Could you check a few things on this drawing? It's one solid part, dimensions in mm from its lowest x, y, z. Give positions to 0.01 mm unless a question says otherwise; leave off trailing zeros. Write each loop counter-clockwise with the first axis right and the second up, starting at its lowest first coordinate (ties: lowest second). Pieces come first, ordered by that corner, then holes. Notation, with made-up numbers: M -26,9.25 L 23,9.25 A18 cw 23,27.25 Z; hole C 42.5,88 d8. An arc over 180 degrees is marked long. Write each question's results on one line, items separated by ' | '.
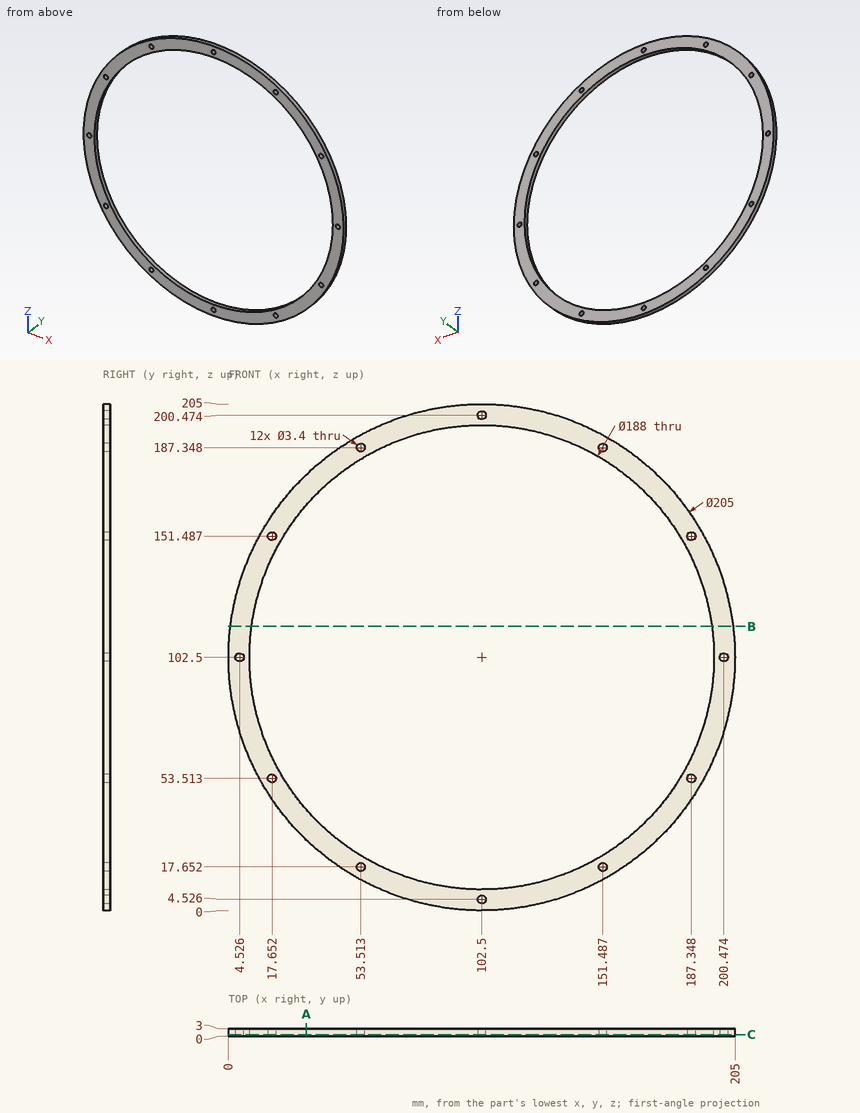
Item 1: I want a section at C-C, the plane y = 0.55. Give the number of separate pieces and of enclosed holes in the cut face, and give its area (3 significant figures).
Geometry says:
separate pieces: 1 | enclosed holes: 13 | area: 5,140 mm2
Item 2: If I drill on line 1 (X direction, y = 2.65, z = 102); line 2 (Z direction, x = 101.5, y = 1.8) (3 decimals); line 3 (X direction, y = 1.35, z = 16.5), over which ranges is the centre line in solid material (lowest first)? Write a range as from..to.
Geometry says:
line 1: x = 0..2.9, 6.15..8.5, 196.5..198.85, 202.1..205 | line 2: z = 0.005..3.151, 5.901..8.505, 196.495..199.099, 201.849..204.995 | line 3: x = 46.73..52.26, 54.76..64.55, 140.45..150.24, 152.74..158.27
Item 3: I want a section at A-A, the plane x = 31.5. Please give me the cut outline in (y, z).
Geometry says:
outline: M 0,28.57 L 3,28.57 L 3,40.9 L 0,40.9 Z; M 0,164.1 L 3,164.1 L 3,176.43 L 0,176.43 Z
Item 4: I want a section at B-B, the plane z = 115. Please give me the cut outline in (x, y) (3 decimals), and give its area (3 significant figures).
Geometry says:
outline: M 0.765,0 L 9.335,0 L 9.335,3 L 0.765,3 Z; M 195.665,0 L 204.235,0 L 204.235,3 L 195.665,3 Z | area: 51.4 mm2
Item 5: I'm going to push a flat-ended pin straight in: pin 1 (2 mm diameter, centred on x = 102.5, z = 4.526, fed in from +Y). Where does the tip first touch, or does it pass through?
Geometry says:
pin 1: passes through
